Here's how the part is built. I have some questions about the finished solid (model axes, mm). Round coordinates to 2 decimals unless told otherwise and drop trailing zeros. Order: outer loops, then holes, each group sorted by start corner. A loop starts at its lowest first (then second) coordinate and runs counter-clockwise, first axis right, second up. Notation, with made-up numbers: (-33, 86.25) - (8, 86.25) arc R20 ccw to (8, 100.25) - close; hole circle Ø4 at (9.5, -8). An arc over 180 degrees is marked (long way). One line per item, written item: value.
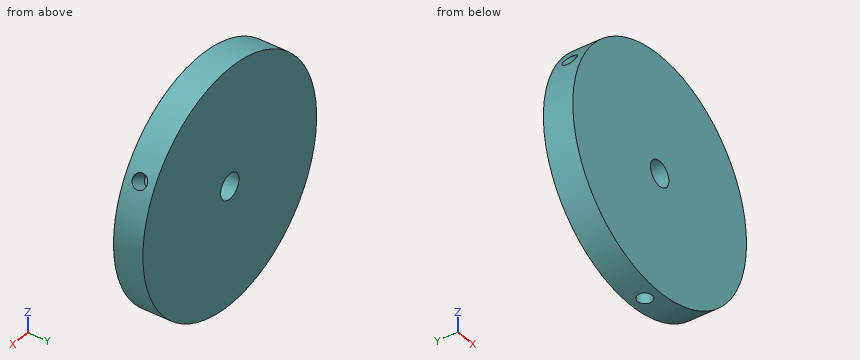
from build123d import *

# Parameters (mm, degrees)
SKETCH1_R           = 38.354
BOSS_EXTRUDE1_DEPTH = 9.525
SKETCH4_R           = 2.3749
CUT_EXTRUDE2_DEPTH  = 6.35
CIRPATTERN1_COUNT   = 3
SKETCH6_R           = 4.064
CUT_EXTRUDE4_DEPTH  = 10.5250001


with BuildPart() as part:
    # Sketch1 → Boss-Extrude1 (new body)
    with BuildSketch(Plane(origin=(0, 0, 0), x_dir=(1, 0, 0), z_dir=(0, 1, 0))):
        Circle(SKETCH1_R)
    extrude(amount=BOSS_EXTRUDE1_DEPTH)

    # Sketch4 → Cut-Extrude2 (cut)
    with BuildSketch(Plane(origin=(-33.215538337, 0, 19.177), x_dir=(0, -1, 0), z_dir=(-0.866025404, 0, 0.5))):
        with Locations((-4.7625, 0)):
            Circle(SKETCH4_R)
    cut_extrude2 = extrude(amount=-CUT_EXTRUDE2_DEPTH, mode=Mode.SUBTRACT)

    # CirPattern1: Cut-Extrude2 ×3 about axis
    cirpattern1_axis = Axis((0, 0, 0), (0, 1, 0))
    for i in range(1, CIRPATTERN1_COUNT):
        add(cut_extrude2.rotate(cirpattern1_axis, i * 360 / CIRPATTERN1_COUNT), mode=Mode.SUBTRACT)

    # Sketch6 → Cut-Extrude4 (cut, through all)
    with BuildSketch(Plane(origin=(0, 9.525, 0), x_dir=(1, 0, 0), z_dir=(0, 1, 0))):
        Circle(SKETCH6_R)
    extrude(amount=-CUT_EXTRUDE4_DEPTH, mode=Mode.SUBTRACT)


solid = part.part
Q1. Will these pins go through, and if not, where does the flat tip stop? pin 1 (1 mm diameter, centred on x = -9.5, y = 1.5, fed in from +Z); pin 2 (1 mm diameter, centred on y = 7, z = -12, fed in from +X); pin 3 (3 mm diameter, centred on x = -8.5, y = 5.5, fed in from -Z).
Results list:
pin 1: z = 37.28
pin 2: x = 36.59
pin 3: z = -37.71
Q2. If I drill on line 1 along Z through (x, y) = (0, 4.5); line 2 along Z through (x, y) = (0, 7.75); line 3 along Y through (x, z) = (0, -33.5) (3 decimals), over which ranges is the centre line in solid material (lowest first)?
Results list:
line 1: -32 to -4.06, 4.06 to 38.35
line 2: -38.35 to -4.06, 4.06 to 38.35
line 3: 0 to 2.388, 7.137 to 9.525
Q3. If we section it at A-A, the plane x = 0: Please give me the cut outline in (y, z) (3 decimals).
Results list:
outline: (0, -38.354) - (2.388, -38.354) - (2.388, -32.004) - (7.137, -32.004) - (7.137, -38.354) - (9.525, -38.354) - (9.525, -4.064) - (0, -4.064) - close; (0, 4.064) - (9.525, 4.064) - (9.525, 38.354) - (0, 38.354) - close
Q4. If we section it at C-C, the plane y = 5.75: Please give me the cut outline in (x, z), then the cut area to 3 significant figures.
Results list:
outline: (-34.24, 17.28) arc R38.35 ccw to (-2.16, -38.29) - (-2.16, -32) - (2.16, -32) - (2.16, -38.29) arc R38.35 ccw to (34.24, 17.28) - (28.8, 14.13) - (26.64, 17.87) - (32.08, 21.02) arc R38.35 ccw to (-32.08, 21.02) - (-26.64, 17.87) - (-28.8, 14.13) - close; hole circle Ø8.13 at (0, 0)
area: 4,490 mm²
Q5. If we section it at D-D, the plane x = 15: Please give me the cut outline in (y, z) (3 decimals), then the cut area to 3 significant figures.
Results list:
outline: (0, -35.299) - (9.525, -35.299) - (9.525, 35.299) - (0, 35.299) - close
area: 672 mm²
Q6. If we section it at B-B, the plane z = 0: Please give me the cut outline in (x, y) (3 decimals).
Results list:
outline: (-38.354, 0) - (-4.064, 0) - (-4.064, 9.525) - (-38.354, 9.525) - close; (4.064, 0) - (38.354, 0) - (38.354, 9.525) - (4.064, 9.525) - close
